Drawing for the job (mm, zero at the part's lowest x, y, z). Give positions to 0.01 mm unless a question says otherwise; leave off trailing zeros. Loops run counter-clockwise (first coordinate to the right, second up) from the corner with the lowest first, then second, coordinate; pieces in that order, holes last. Notation, with made-up numbers: (11.25, 20.5) -> (41.25, 20.5) arc R23 ccw to (41.25, 46.5) -> close; hole circle Ø9 at (-13, 71.5). An arc over 180 degrees is marked (long way). Answer in a Markdown table with one row per item. Add a question column.
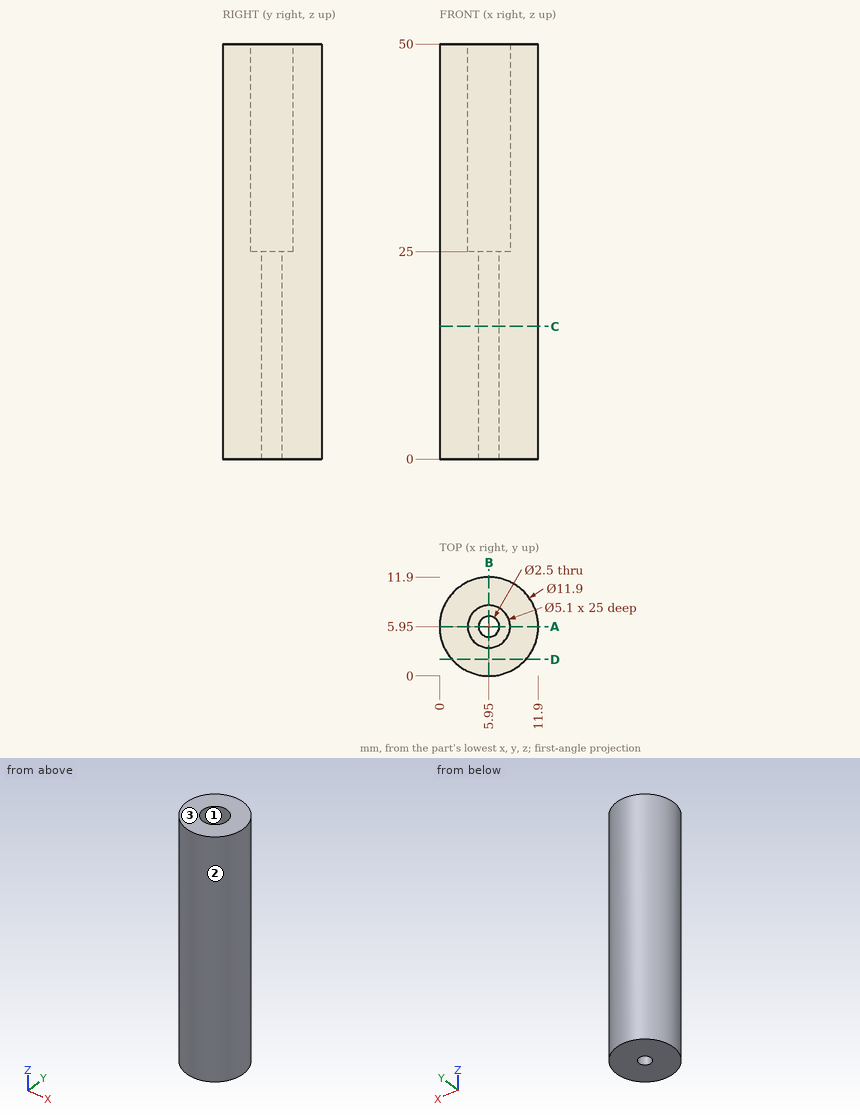
(1) Saw through at D-D, the plane y = 2. List the corners of the cut face in (x, z), then the cut area to 3 significant figures.
(2) Saw through at C-C, the plane z = 16. List the corners of the cut face in (x, y).
(3) Wall check: line 1 along Y through (x, z) = (5.95, 10.5); line 2 along X through (y, z) = (6, 26); line 3 along Y through (x, z) = (6.5, 47). Give the ranges that are in metal, low to high. Write a range as from..to.
(4) Saw through at A-A, the plane y = 5.95. List the corners of the cut face in (x, z), then the cut area to 3 significant figures.
(5) Flat gauge pin, fed straight in: pin 1 Ø1.5 at (x, y) = (5.95, 5.95) entering from -Z. Where does the tip first touch, or does it go through?
(6) Two-plate mould, pull along X, no slides. Class the marked faces 1, 2 and 3: released by +X, released by -X, zero draft, split by the parting line, or undercut.
Worked answers:
| question | item | result |
|---|---|---|
| 1 | outline | (1.5, 0) -> (10.4, 0) -> (10.4, 50) -> (1.5, 50) -> close |
| 1 | area | 445 mm^2 |
| 2 | outline | circle Ø11.9 at (5.95, 5.95); hole circle Ø2.5 at (5.95, 5.95) |
| 3 | line 1 | 0..4.7, 7.2..11.9 |
| 3 | line 2 | 0..3.4, 8.5..11.9 |
| 3 | line 3 | 0.03..3.46, 8.44..11.87 |
| 4 | outline | (0, 0) -> (4.7, 0) -> (4.7, 25) -> (3.4, 25) -> (3.4, 50) -> (0, 50) -> close; (7.2, 0) -> (11.9, 0) -> (11.9, 50) -> (8.5, 50) -> (8.5, 25) -> (7.2, 25) -> close |
| 4 | area | 405 mm^2 |
| 5 | pin 1 | through |
| 6 | face 1 | undercut |
| 6 | face 2 | split by the parting line |
| 6 | face 3 | zero draft |
